Build history of the part. All positions in model axes, mm. Face numbers are marked on the shaded views. A direction names the side the tool comes from. Coordinates: 2 decimals unless noted, no trailing zeros. Loops run counter-clockwise (first coordinate to the right, second up) from the corner with the lowest first, then second, coordinate; pieces in that order, holes last.
(1) Slice it at B-B (z = 0). Give the cut face in (x, y), and give its area (3 significant figures).
(2) Slice it at C-C (y = -20). Give the cut face in (x, z), and give its area (3 significant figures).
(3) Wall check: L1, parallel to Y at x = 35, z = 1; L2, parallel to Y at x = -69.5, z = -10; L3, parallel to Z at x = 44, y = -21. Give the ranges that are in metal, low to high.
(4) Two-plate mould, pull along Y, no slides. Class the marked faces 3, 4 and 5: pulls with the +Y half, pulls with the -Y half, needs draft (parallel to the pull), parting line crosses it, or undercut.
(5) Slice it at A-A (x = 7). Give the cut face in (y, z), and give its area (3 significant figures).
(6) Flat gauge pins, fed straight in: P1, Ø11, axis at y = -14.5, z = 3.5, coming from the -X side; P2, Ø1, axis at x = 53, y = -28.5, coming from the +Z side; P3, Ø3, axis at x = -28.5, y = -16, coming from the -Z side. Where does each tip first touch, or does it go through?
(7) Slice it at D-D (x = -56). Give the cut face in (y, z), and give its area (3 significant figures).
(8) Tool access for the marked faces 1 and 2: list every direction of +Z, -Z, +X, -X, +Y, -Y with a clear straight run to the whole face (end or side of a thin tool).
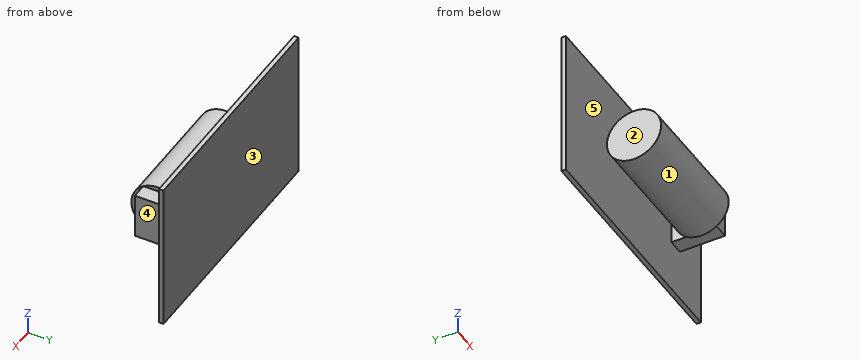
from build123d import *

# Parameters (mm, degrees)
SKETCH1_W           = 160
SKETCH1_H           = 100
BOSS_EXTRUDE1_DEPTH = 3
SKETCH2_W           = 10
SKETCH2_H           = 30
BOSS_EXTRUDE2_DEPTH = 30
SKETCH3_R           = 18
BOSS_EXTRUDE3_DEPTH = 80


with BuildPart() as part:
    # Sketch1 → Boss-Extrude1 (new body)
    with BuildSketch(Plane(origin=(0, 0, 0), x_dir=(1, 0, 0), z_dir=(0, 1, 0))):
        Rectangle(SKETCH1_W, SKETCH1_H)
    extrude(amount=BOSS_EXTRUDE1_DEPTH)

    # Sketch2 → Boss-Extrude2 (add)
    with BuildSketch(Plane(origin=(0, 0, 0), x_dir=(1, 0, 0), z_dir=(0, 1, 0))):
        with Locations((50, 0)):
            Rectangle(SKETCH2_W, SKETCH2_H)
    extrude(amount=-BOSS_EXTRUDE2_DEPTH)

    # Sketch3 → Boss-Extrude3 (add)
    with BuildSketch(Plane.ZY.offset(-45)):
        with Locations(Location((0, -20, 0), (0, 0, 146.442690238))):
            Circle(SKETCH3_R)
    extrude(amount=BOSS_EXTRUDE3_DEPTH)


solid = part.part
Response values:
1. outline: (-80, 0) - (45, 0) - (45, -2) - (-35, -2) - (-35, -38) - (45, -38) - (45, -30) - (55, -30) - (55, 0) - (80, 0) - (80, 3) - (-80, 3) - close
1. area: 3,660 mm2
2. outline: (-35, -18) - (45, -18) - (45, -15) - (55, -15) - (55, 15) - (45, 15) - (45, 18) - (-35, 18) - close
2. area: 3,180 mm2
3. L1: y = -37.97 to -2.03, 0 to 3
3. L2: y = 0 to 3
3. L3: z = -17.97 to 17.97
4. face 3: pulls with the +Y half
4. face 4: needs draft
4. face 5: undercut
5. outline: circle Ø36 at (-20, 0); (0, -50) - (3, -50) - (3, 50) - (0, 50) - close
5. area: 1,320 mm2
6. P1: stops at x = -35
6. P2: stops at z = 15
6. P3: stops at z = -17.83
7. outline: (0, -50) - (3, -50) - (3, 50) - (0, 50) - close
7. area: 300 mm2
8. face 1: -X
8. face 2: +Z, -Z, -X, -Y
